Autodesk Inventor part; units mm, degrees
ref_plane "YZ Plane" through (0, 0, 0) normal (1, 0, 0) x (0, 1, 0)
ref_plane "XZ Plane" through (0, 0, 0) normal (0, 1, 0) x (-1, 0, 0)
ref_plane "XY Plane" through (0, 0, 0) normal (0, 0, 1) x (1, 0, 0)
sketch "Эскиз1" plane through (0, 0, 0) normal (0, 0, 1) x (1, 0, 0)
  line L0 (-9.0572, 59.3125) -> (-55.8947, -21.8125)
  line L1 (-46.8375, -37.5) -> (46.8375, -37.5)
  line L2 (9.0572, 59.3125) -> (55.8947, -21.8125)
  arc A0 (9.0572, 59.3125) -> (-9.0572, 59.3125) centre (0, 0) ccw
  arc A1 (-55.8947, -21.8125) -> (-46.8375, -37.5) centre (0, 0) ccw
  arc A2 (46.8375, -37.5) -> (55.8947, -21.8125) centre (0, 0) ccw
  circle A3 centre (0, 47.5) radius 6
  circle A4 centre (41.1362, -23.75) radius 6
  circle A5 centre (-41.1362, -23.75) radius 6
  point P0 (51.9615, -30)
  dimension "d3" = 12
  dimension "d4" = 12
  dimension "d5" = 12
  dimension "d7" = 47.5
  dimension "d8" = 41.1362
  dimension "d9" = 41.1362
  dimension "d10" = 13.75
  dimension "d11" = 13.75
  dimension "d12" = 13.75
extrude "Выдавливание1" add sketch "Эскиз1" along normal blind 15
sketch "Эскиз2" plane through (0, 0, 15) normal (0, 0, 1) x (1, 0, 0)
  circle A0 centre (0, 0) radius 35
  dimension "d15" = 70
extrude "Выдавливание2" add sketch "Эскиз2" along normal blind 19
sketch "Эскиз4" plane through (0, 0, 0) normal (0, 1, 0) x (-1, 0, 0)
  line L0 (35, 34) -> (-35, 34)
  line L1 (30.9218, 34) -> (35, 26.9363)
  line L2 (35, 15) -> (35, 34)
  line L3 (30.9218, 34) -> (35, 34)
  line L4 (0, -6.8) -> (0, 40.8)
  point P0 (0, 0)
  dimension "d21" = 30
revolve "Вращение1" cut sketch "Эскиз4" angle 360 about axis through (0, 0, -10) along (0, 0, 1)
sketch "Эскиз5" plane through (0, 0, 34) normal (0, 0, 1) x (1, 0, 0)
  circle A0 centre (0, 0) radius 16.5
  dimension "d23" = 33
extrude "Выдавливание3" add sketch "Эскиз5" along normal blind 5
sketch "Эскиз6" plane through (0, 0, 39) normal (0, 0, 1) x (1, 0, 0)
  circle A0 centre (0, 0) radius 11.25
  dimension "d26" = 22.5
extrude "Выдавливание4" add sketch "Эскиз6" along normal blind 7
sketch "Эскиз7" plane through (0, 0, 46) normal (0, 0, 1) x (1, 0, 0)
  circle A0 centre (0, 0) radius 13.5
  dimension "d29" = 27
extrude "Выдавливание5" add sketch "Эскиз7" along normal blind 24
sketch "Эскиз8" plane through (0, 0, 0) normal (0, 0, -1) x (-1, 0, 0)
  circle A0 centre (0, 0) radius 27
  dimension "d32" = 54
extrude "Выдавливание6" cut sketch "Эскиз8" against normal blind 10
sketch "Эскиз15" plane through (0, 0, 10) normal (0, 0, -1) x (-1, 0, 0)
  circle A0 centre (0, 0) radius 14
  dimension "d54" = 28
extrude "Выдавливание11" cut sketch "Эскиз15" against normal blind 21
chamfer "Фаска1" distance 6 angle 45 1 edges at (14, 0, 10)
sketch "Эскиз16" plane through (0, 0, 31) normal (0, 0, -1) x (-1, 0, 0)
  circle A0 centre (0, 0) radius 6
  dimension "d60" = 12
extrude "Выдавливание12" cut sketch "Эскиз16" against normal blind 39
thread "Резьба1"
fillet "Сопряжение1" radius 1.6 1 edges at (-11.25, 0, 39)
chamfer "Фаска2" distance 2.25 angle 45 1 edges at (-11.25, 0, 46)
fillet "Сопряжение2" radius 1 1 edges at (-11.25, 0, 43.7501)
chamfer "Фаска3" distance 2.5 angle 45 1 edges at (-13.5, 0, 70)
chamfer "Фаска4" distance 1 angle 45 1 edges at (6, 0, 70)
Work out the finished part from the listing and answer in its coordinate system (mm). A direction names the side the tool comes from. Round coordinates to 2 decimals unless told otherwise and drop trailing zeros. Write each loop counter-clockwise with the first axis right and the second up, starting at its lowest first coordinate (ties: lowest second). Pieces come first, ordered by that corner, then holes. Notation, with made-up numbers: (28, 33.5) - (78, 33.5) arc R22 ccw to (78, 68.5) - close; hole circle Ø1 at (23, 12.5). An arc over 180 degrees is marked (long way). Return JSON: item names as keys, results as strings. Group by question number.
Q1. The part is cut by section A-A on y = 49.5. Write down the section's boundary in (x, z), then the cut area to 3 significant figures.
Q2. The mould has two halves that part along X. Classify faces 1 (the cylindrical face through (-51.9, -30.11, 7.4)), 2 (the flat face through (-21, -17.4, 0)), 3 (the cylindrical face through (5.85, -26.36, 4.93)), 4 (the cylindrical face through (5.19, 9.98, 41.95)): released by +X, released by -X, zero draft, split by the parting line, or undercut.
Q3. The part is cut by section C-C on x = 0. Count the separate pieces of the cut face and the enclosed holes in it, then the cut area to 3 significant figures.
Q4. For faces 5 (the flat face through (-1, -37.5, 7)), 6 (the cylindrical face through (-28, 21, 21)), 7 (the cylindrical face through (-12.932, -5.362, 23.395)), 8 (the conical face through (-2.53, -11.39, 44.17)), determine the directions among +Z, -Z, +X, -X, +Y, -Y from which every point of the face is accessible in a straight line to the end or side of a thin tool.
Q5. The part is cut by section B-B on z = 22.5. Write down the section's boundary in (x, y), then the cut area to 3 significant figures.
Q6. Each of these flat-tipped pins is pushed along its axis until it touches: pin 1 Ø6 at (x, z) = (-5.5, 14.5) entering from +Y; pin 2 Ø14 at (x, y) = (-4.5, -2) entering from -Z. Where does it stop, or does it pass through?
Q7. Find the intervals of material crossed by L1, parallel to Z at x = -46, y = -18.5; L2, parallel to Y at x = 0, z = 41; L3, parallel to Z at x = -11, y = 22, in increasing order.
Solved:
{
 "1": {"outline": "(-14.72, 0) - (-5.66, 0) - (-5.66, 15) - (-14.72, 15) - close; (5.66, 0) - (14.72, 0) - (14.72, 15) - (5.66, 15) - close", "area": "272 mm²"},
 "2": {"face 1": "released by -X", "face 2": "zero draft", "face 3": "undercut", "face 4": "split by the parting line"},
 "3": {"separate pieces": "3", "enclosed holes": "0", "area": "1,920 mm²"},
 "4": {"face 5": "+Z, -Z, +X, -X, -Y", "face 6": "+Z", "face 7": "-Z", "face 8": "none"},
 "5": {"outline": "circle Ø70 at (0, 0); hole circle Ø28 at (0, 0)", "area": "3,230 mm²"},
 "6": {"pin 1": "y = 59.95", "pin 2": "z = 31"},
 "7": {"L1": "0 to 15", "L2": "-11.25 to -6, 6 to 11.25", "L3": "10 to 34"}
}
